from build123d import *

# Parameters (mm, degrees)
SKETCH_1_R          = 4
EXTRUDE_1_DEPTH     = 5
SKETCH_2_R          = 2
CUT_EXTRUDE_1_DEPTH = 8.549834435
M3X0_5_1_REACH      = 11.486
M3X0_5_1_BORE_R     = 1.5


with BuildPart() as part:
    # ｽｹｯﾁ1 → ﾎﾞｽ - 押し出し1 (new body)
    with BuildSketch(Plane.XY):
        Circle(SKETCH_1_R)
    extrude(amount=EXTRUDE_1_DEPTH)

    # ｽｹｯﾁ2 → ｶｯﾄ - 押し出し1 (cut, through all)
    with BuildSketch(Plane.XY.offset(5)):
        Circle(SKETCH_2_R)
    extrude(amount=-CUT_EXTRUDE_1_DEPTH, mode=Mode.SUBTRACT)

    # M3x0.5 ねじ穴1 bore (on position points) → M3x0.5 ねじ穴1 (cut, up to next)
    with BuildSketch(Plane(origin=(0.497313961, 3.968964452, 2.5), x_dir=(0.992241113083, -0.124328490328, 0), z_dir=(0.124328490328, 0.992241113083, 0)), mode=Mode.PRIVATE) as m3x0_5_1_sk1:
        Circle(M3X0_5_1_BORE_R)
    m3x0_5_1_tool1 = extrude(m3x0_5_1_sk1.sketch, amount=-M3X0_5_1_REACH, mode=Mode.PRIVATE) & part.part
    add(m3x0_5_1_tool1.solids().sort_by_distance((0.497314, 3.968964, 2.5))[0], mode=Mode.SUBTRACT)


solid = part.part
Geometry check sheet. Reference: the model listing, model coordinates, mm. Round coordinates to 2 decimals unless told otherwise and drop trailing zeros. Write each loop counter-clockwise with the first axis right and the second up, starting at its lowest first coordinate (ties: lowest second). Pieces come first, ordered by that corner, then holes. Notation, with made-up numbers: (-9, -4) -> (0, -4) arc R9 ccw to (0, 10) -> close; hole circle Ø8 at (-9.5, -31). An arc over 180 degrees is marked (long way). One line per item, written item: value. Start each with the question number.
(1) Scan lines: line 1 (Y direction, x = 0, z = 3.25); line 2 (Y direction, x = 1.75, z = 1); line 3 (X direction, y = 1.5, z = 2.8). Record each from-to range of solid material in increasing order. Write a range as [from, to].
(2) Cross-section at A-A, the plane y = 0. Record the cut outline in (x, z), and give its area (3 significant figures).
(3) Cross-section at B-B, the plane x = -1.5. Record the cut outline in (y, z), and give its area (3 significant figures).
(4) Cross-section at C-C, the plane z = 0.4. Record the cut outline in (x, y), and give its area (3 significant figures).
(5) Go/stop test with flat-tipped pins: pin 1 Ø1.5 at (x, z) = (3, 4) entering from -Y; pin 2 Ø2 at (x, z) = (-2, 2) entering from +Y; pin 3 Ø3 at (x, y) = (0, 0) entering from -Z. Record where each tip stops, or that it passes through.
(6) Draft check along X on faces 1 (the cylindrical face through (1.753, 2.482, 2.049)), 2 (the flat face through (-2, -1, 0)), 3 (the cylindrical face through (-0.867, -3.905, 2.465)). Enter one of: +X half, -X half, draft (parallel to the pull), parting line (faces both ways), or undercut.
(7) Cross-section at D-D, the plane x = 0.5. Give the number of separate pieces and of enclosed holes in the cut face, and give its area (3 significant figures).
Answer:
1. line 1: [-4, -2]
1. line 2: [-3.6, -0.97], [0.97, 3.6]
1. line 3: [-3.71, -1.32], [1.67, 3.71]
2. outline: (-4, 0) -> (-2, 0) -> (-2, 5) -> (-4, 5) -> close; (2, 0) -> (4, 0) -> (4, 5) -> (2, 5) -> close
2. area: 20.0 mm²
3. outline: (-3.71, 0) -> (-1.32, 0) -> (-1.32, 5) -> (-3.71, 5) -> close; (1.32, 0) -> (3.71, 0) -> (3.71, 5) -> (1.32, 5) -> close
3. area: 23.9 mm²
4. outline: circle Ø8 at (0, 0); hole circle Ø4 at (0, 0)
4. area: 37.7 mm²
5. pin 1: y = -3.31
5. pin 2: y = 3.87
5. pin 3: through
6. face 1: undercut
6. face 2: draft
6. face 3: parting line
7. separate pieces: 3
7. enclosed holes: 0
7. area: 14.3 mm²
